Print and shaded views of the part. All mm, measured from the part's lowest x, y and z. Round coordinates to 2 decimals unless told otherwise and drop trailing zeros. Write each loop counter-clockwise with the first axis right and the second up, starting at its lowest first coordinate (ties: lowest second). Pieces come first, ordered by that corner, then holes. Notation, with made-up numbers: (81.25, 54) - (113.25, 54) arc R18 ccw to (113.25, 79) - close; hole circle Ø7 at (-13, 48). An arc over 180 degrees is marked (long way). Put each result on its own line as item: value. Start each with the question number.
Item 1: Cut at A-A (x = 100). Give the cut face in (y, z).
Item 2: Drill centre lines: line 1 (Y direction, x = 20, z = 8.75); line 2 (X direction, y = 155, z = 5.5); line 3 (Y direction, x = 102, z = 1.75). Where is each one in solid material? Low to high. Write a range as from..to.
Item 3: Cut at B-B (y = 35). Give the cut face in (x, z), and give its area (3 significant figures).
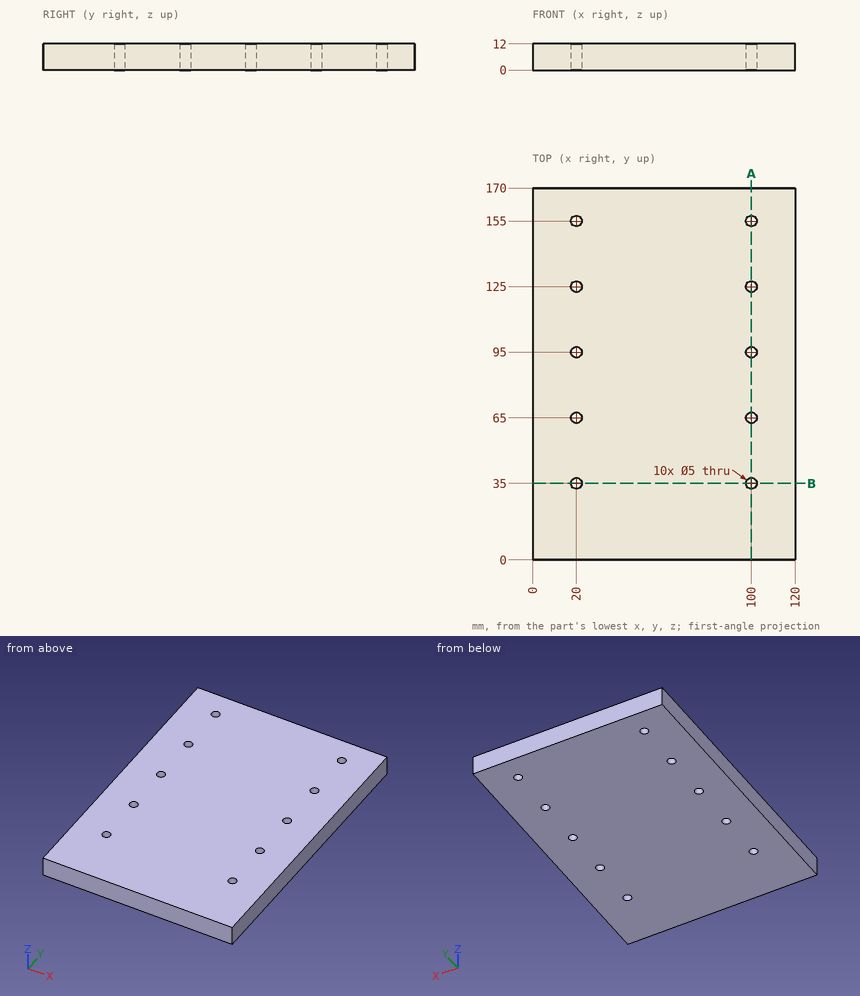
Output values:
1. outline: (0, 0) - (32.5, 0) - (32.5, 12) - (0, 12) - close; (37.5, 0) - (62.5, 0) - (62.5, 12) - (37.5, 12) - close; (67.5, 0) - (92.5, 0) - (92.5, 12) - (67.5, 12) - close; (97.5, 0) - (122.5, 0) - (122.5, 12) - (97.5, 12) - close; (127.5, 0) - (152.5, 0) - (152.5, 12) - (127.5, 12) - close; (157.5, 0) - (170, 0) - (170, 12) - (157.5, 12) - close
2. line 1: 0..32.5, 37.5..62.5, 67.5..92.5, 97.5..122.5, 127.5..152.5, 157.5..170
2. line 2: 0..17.5, 22.5..97.5, 102.5..120
2. line 3: 0..33.5, 36.5..63.5, 66.5..93.5, 96.5..123.5, 126.5..153.5, 156.5..170
3. outline: (0, 0) - (17.5, 0) - (17.5, 12) - (0, 12) - close; (22.5, 0) - (97.5, 0) - (97.5, 12) - (22.5, 12) - close; (102.5, 0) - (120, 0) - (120, 12) - (102.5, 12) - close
3. area: 1,320 mm2
